Model file for the job. Use its own axes, mm. Face numbers are marked on the shaded views. Coordinates: 2 decimals unless noted, no trailing zeros. Order: outer loops, then holes, each group sorted by start corner. A loop starts at its lowest first (then second) coordinate and runs counter-clockwise, first axis right, second up. Notation, with made-up numbers: M -33,6 L -20,6 A12 cw -20,20 Z; hole C 12.5,-26 d9. An arc over 180 degrees is marked long. Return JSON: item names as keys, results as strings.
```python
from build123d import *

# Parameters (mm, degrees)
SKETCH1_W        = 10
SKETCH1_H        = 25
DIAMETER_HOLE1_D = 6.5
DIAMETER_HOLE2_D = 6.5


with BuildPart() as part:
    # Sketch1 → Revolve1 (revolve)
    with BuildSketch(Plane.XY, mode=Mode.PRIVATE) as revolve1_sk:
        with Locations((5, 22.5)):
            Rectangle(SKETCH1_W, SKETCH1_H)
    revolve(revolve1_sk.sketch.rotate(Axis((0, 0, 0), (1, 0, 0)), 90), axis=Axis((0, 0, 0), (1, 0, 0)))

    # Diameter Hole1 (through all)
    with Locations(Plane(origin=(10, 0, 0), x_dir=(0, 0, -1), z_dir=(1, 0, 0))):
        with Locations((-16, 0), (0, 16), (16, 0), (0, -16)):
            Hole(DIAMETER_HOLE1_D / 2)

    # Diameter Hole2 (through all)
    with Locations(Plane(origin=(10, 0, 0), x_dir=(0, 0, -1), z_dir=(1, 0, 0))):
        with Locations((-12.02081528, -12.02081528), (12.02081528, 12.02081528)):
            Hole(DIAMETER_HOLE2_D / 2)


solid = part.part
```
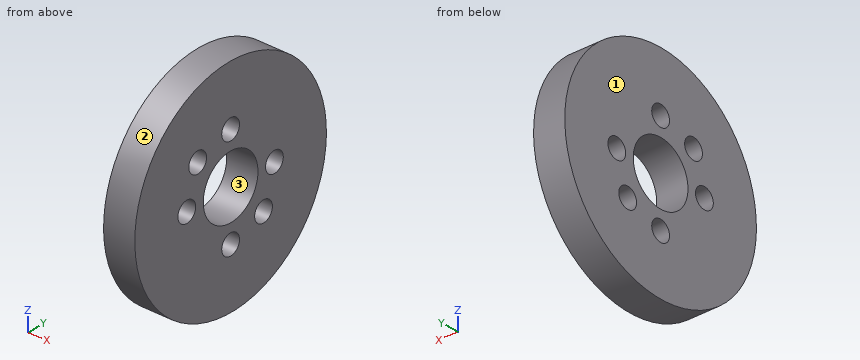
Item 1: Pull direction Y, two halves, no side cores. Call the marked faces 1, 2 and 3: +Y half, -Y half, draft (parallel to the pull), parting line (faces both ways), or undercut.
Check result:
{"face 1": "draft", "face 2": "parting line", "face 3": "undercut"}
Item 2: Saw through at A-A (y = 1.5). Write the cut outline in (x, z), and give its area (3 significant figures).
Check result:
{"outline": "M 0,-34.97 L 10,-34.97 L 10,-18.88 L 0,-18.88 Z; M 0,-13.12 L 10,-13.12 L 10,-9.89 L 0,-9.89 Z; M 0,9.89 L 10,9.89 L 10,13.12 L 0,13.12 Z; M 0,18.88 L 10,18.88 L 10,34.97 L 0,34.97 Z", "area": "386 mm2"}
Item 3: Saw through at B-B (x = 3.25). Write the cut outline in (y, z), and give its area (3 significant figures).
Check result:
{"outline": "C 0,0 d70; hole C -16,0 d6.5; hole C -12.02,12.02 d6.5; hole C 0,0 d20; hole C 0,-16 d6.5; hole C 0,16 d6.5; hole C 12.02,-12.02 d6.5; hole C 16,0 d6.5", "area": "3,340 mm2"}
Item 4: Saw through at D-D (y = 20.5). Write the cut outline in (x, z), and give its area (3 significant figures).
Check result:
{"outline": "M 0,-28.37 L 10,-28.37 L 10,28.37 L 0,28.37 Z", "area": "567 mm2"}
Item 5: Wall check: line 1 (Y direction, x = 5.5, z = 0); line 2 (Z direction, x = 1, y = -14); line 3 (Y direction, x = 3.5, z = 3). Give the ranges that are in metal, low to high.
Check result:
{"line 1": "y = -35 to -19.25, -12.75 to -10, 10 to 12.75, 19.25 to 35", "line 2": "z = -32.08 to -2.56, 2.56 to 9.44, 14.6 to 32.08", "line 3": "y = -34.87 to -17.25, -14.75 to -9.54, 9.54 to 14.75, 17.25 to 34.87"}
Item 6: Saw through at C-C (z = 26). Write the cut outline in (x, y), and give its area (3 significant figures).
Check result:
{"outline": "M 0,-23.43 L 10,-23.43 L 10,23.43 L 0,23.43 Z", "area": "469 mm2"}
Item 7: Drop flat-ended pins along their axis: pin 1 Ø1 at (x, y) = (6, 22.5) entering from +Z; pin 2 Ø3 at (x, z) = (2.5, 13) entering from +Y; pin 3 Ø5 at (x, z) = (2.5, -13.5) entering from +Y. Give the stop position or say it passes through.
Check result:
{"pin 1": "stops at z = 27.22", "pin 2": "stops at y = 33.06", "pin 3": "stops at y = 33.23"}
